Answer from the drawing. Dimensions are ordinates in mm from the lowest x, y and z of the part. Give positions to 0.01 mm unless a question says otherwise; leave off trailing zeros. Write each loop counter-clockwise with the first axis right and the second up, starting at its lowest first coordinate (ties: lowest second). Pieces come first, ordered by that corner, then holes. Notation, with made-up numbers: (56, 37.5) -> (106, 37.5) arc R23 ccw to (106, 76.5) -> close; hole circle Ø10 at (-34, 64). An arc over 180 degrees is marked (long way). Put each result on its own line as item: value. Start each with the question number.
1) A cutting plane is placed at B-B (x = 84). Write down the section's boundary in (y, z) (1 decimal).
2) A cutting plane is placed at D-D (x = 42). Write down the section's boundary in (y, z) (1 decimal).
3) Flat-ended cylindrical pins translate along their axes: pin 1 Ø1.5 at (x, y) = (28.5, 3) entering from -Z; pin 2 Ø3 at (y, z) = (2.5, 49.5) entering from -X; pin 3 Ø1.5 at (x, y) = (26.5, 2) entering from +Z. Find the tip coordinate at first contact, or state that the pin passes through.
4) Find the intervals of material crossed by line 1 along Z through (x, y) = (48.5, 1.1) (1 decimal); line 2 along X through (y, z) = (2.1, 34) (1 decimal); line 3 along X through (y, z) = (2.5, 29) (1 decimal), in increasing order. Write a range as from..to.
5) A cutting plane is placed at C-C (z = 28). Write down the section's boundary in (x, y), then the cut area to 3 significant figures.
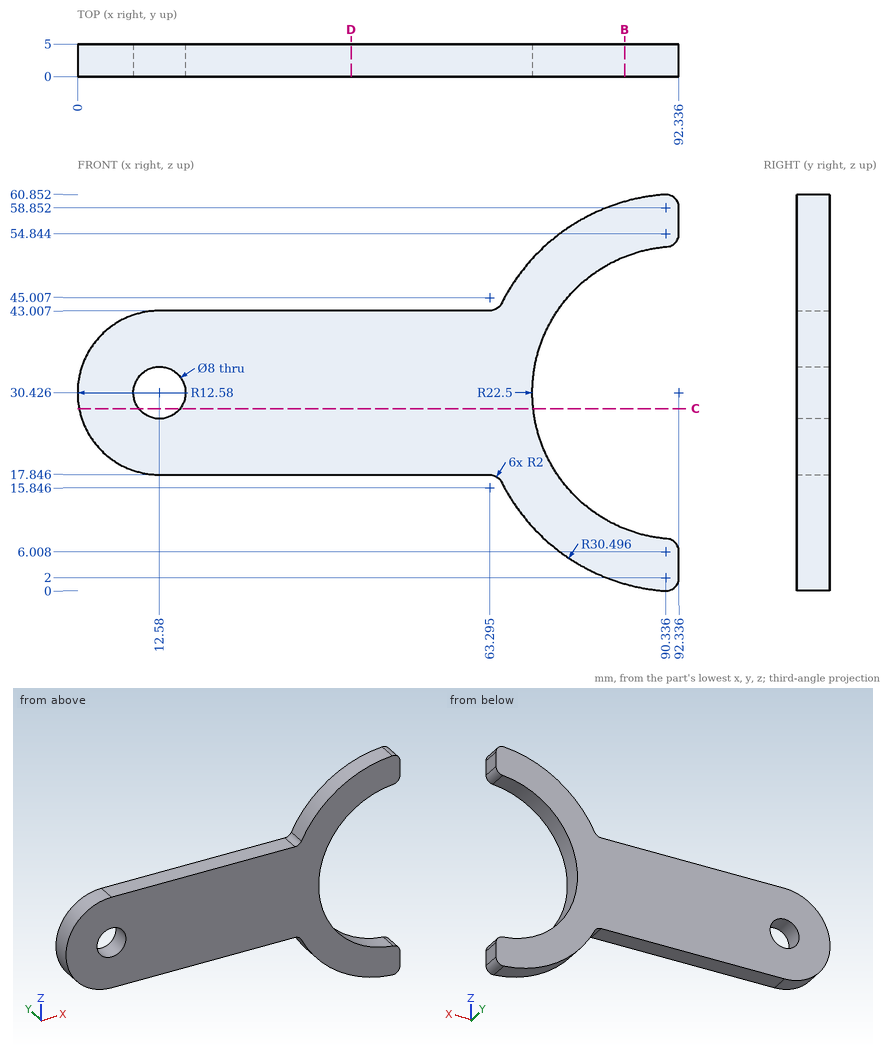
Reply:
1. outline: (0, 1.1) -> (5, 1.1) -> (5, 9.5) -> (0, 9.5) -> close; (0, 51.3) -> (5, 51.3) -> (5, 59.8) -> (0, 59.8) -> close
2. outline: (0, 17.8) -> (5, 17.8) -> (5, 43) -> (0, 43) -> close
3. pin 1: stops at z = 17.85
3. pin 2: stops at x = 67.41
3. pin 3: stops at z = 43.01
4. line 1: z = 17.8..43
4. line 2: x = 0.5..10.8, 14.4..70.1
4. line 3: x = 0.1..8.8, 16.3..69.9
5. outline: (0.24, 0) -> (9.4, 0) -> (9.4, 5) -> (0.24, 5) -> close; (15.76, 0) -> (69.97, 0) -> (69.97, 5) -> (15.76, 5) -> close
5. area: 317 mm2
